Input: part model. Units: mm. Frame: model coordinates. Face numbers are marked on the shaded views. A direction names the side the tool comes from. Coordinates: 2 decimals unless noted, no trailing zeros. Loops run counter-clockwise (first coordinate to the right, second up) from the corner with the lowest first, then second, coordinate; pieces in that order, holes last.
(1) Contact query for flat-ended pins moving along their axis: P1, Ø3, axis at y = -2.5, z = 17, coming from the -X side; P2, Ø0.8, axis at x = -23, z = 16.5, coming from the -Y side; P3, Ø5, axis at x = -8.5, z = 0, coming from the -Y side. Output: stop coordinate, or through.
(2) Section B-B, the plane x = -23. Return loops of the section in (y, z), then the cut area to 3 significant figures.
(3) Line query: L1, parallel to X at y = -4.5, z = -18.5; L2, parallel to Z at x = 0, y = 0.2; L3, parallel to Z at x = -12, y = -3.75. Output: solid intervals per line, ascending.
(4) Section D-D, the plane z = -8.5. Return loops of the section in (x, y), then the cut area to 3 significant figures.
(5) Section C-C, the plane y = -6.25. Return loops of the section in (x, z).
(6) Mould query, pull axis Z, two halves, no side actions, for the marked faces 1, 2 and 3. Classes: released by +Z, released by -Z, zero draft, split by the parting line, or undercut.
(7) Section A-A, the plane z = 17. Return loops of the section in (x, y).
(8) Set-up query: the marked faces 4 and 5. Return all of +Z, -Z, +X, -X, +Y, -Y with unobstructed straight access to the full face (end or side cutting, diameter ignored); none if empty.
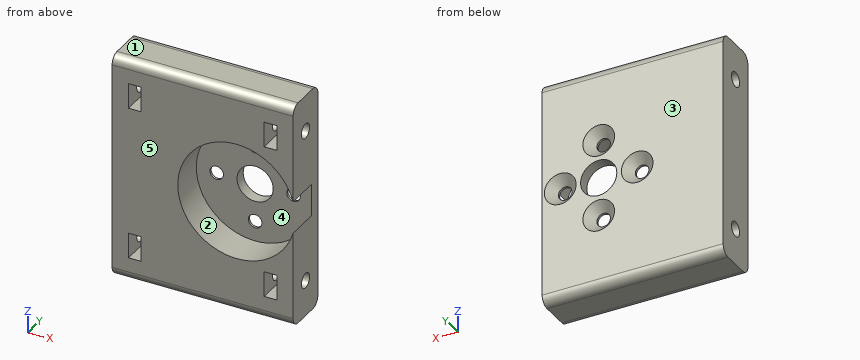
Autodesk Inventor part; units mm, degrees
ref_plane "YZ Plane" through (0, 0, 0) normal (1, 0, 0) x (0, 1, 0)
ref_plane "XZ Plane" through (0, 0, 0) normal (0, 1, 0) x (-1, 0, 0)
ref_plane "XY Plane" through (0, 0, 0) normal (0, 0, 1) x (1, 0, 0)
sketch "Эскиз1" plane through (0, 0, 0) normal (0, 1, 0) x (-1, 0, 0)
  circle A0 centre (0, 0) radius 12.5 construction
  circle A1 centre (0, 0) radius 8.5 construction
  circle A2 centre (8.5, 0) radius 1.5
  circle A3 centre (-8.5, 0) radius 1.5
  circle A4 centre (0, 0) radius 4
  line L0 (27.5, 25) -> (-12.5, 25)
  line L1 (-12.5, 25) -> (-12.5, -25)
  line L2 (-12.5, -25) -> (27.5, -25)
  line L3 (27.5, -25) -> (27.5, 25)
  line L4 (0, -12.5) -> (0, 12.5) construction
  line L5 (-12.5, 0) -> (12.5, 0) construction
  circle A5 centre (0, -8.5) radius 1.5
  circle A6 centre (0, 8.5) radius 1.5
  point P0 (7.5, 25)
  point P1 (7.5, -25)
  dimension "d0" = 25
  dimension "d1" = 17
  dimension "d2" = 3
  dimension "d3" = 3
  dimension "d4" = 8
  dimension "d5" = 40
  dimension "d6" = 50
  dimension "d7" = 25
  dimension "d26" = 25
  dimension "d31" = 90
  dimension "d32" = 90
  dimension "d33" = 3
  dimension "d34" = 3
extrude "Выдавливание1" add sketch "Эскиз1" along normal blind 2.5
sketch "Эскиз2" plane through (0, 0, 0) normal (0, -1, 0) x (1, 0, 0)
  circle A0 centre (0, 0) radius 13
  line L0 (12.5, 25) -> (12.5, -25)
  line L1 (-27.5, 25) -> (12.5, 25)
  line L2 (-27.5, -25) -> (-27.5, 25)
  line L3 (12.5, -25) -> (-27.5, -25)
  circle A1 centre (-8.5, 0) radius 1.5
  circle A2 centre (8.5, 0) radius 1.5
  circle A3 centre (0, 0) radius 4
  point P0 (12.5, -3.5707)
  point P1 (12.5, 3.5707)
  dimension "d10" = 26
extrude "Выдавливание2" add sketch "Эскиз2" along normal blind 7.5 contours A0 L0 L3 L2 L1
fillet "Сопряжение1" radius 2 4 edges at (-7.5, -7.5, -25) (-7.5, 2.5, -25) (-7.5, -7.5, 25) (-7.5, 2.5, 25)
sketch "Эскиз4" plane through (-27.5, -5.5, -25) normal (-1, 0, 0) x (0, 0, 1)
  arc A0 (50, 6) -> (48, 8) centre (48, 6) ccw
  line L0 (2, 8) -> (48, 8)
  arc A1 (2, 8) -> (0, 6) centre (2, 6) ccw
  line L1 (0, 0) -> (0, 6)
  arc A2 (0, 0) -> (2, -2) centre (2, 0) ccw
  line L2 (48, -2) -> (2, -2)
  arc A3 (48, -2) -> (50, 0) centre (48, 0) ccw
  line L3 (50, 0) -> (50, 6)
  circle A4 centre (42, 3) radius 1.65
  circle A5 centre (8, 3) radius 1.65
  point P0 (25, 5.5)
  point P1 (50, 3)
  dimension "d21" = 3.3
  dimension "d22" = 3.3
  dimension "d41" = 5
  dimension "d42" = 34
  dimension "d43" = 8
  dimension "d44" = 5
extrude "Выдавливание4" cut sketch "Эскиз4" against normal through all contours A4 | A5
chamfer "Фаска1" distance 2 angle 45 4 edges at (-7, 2.5, 0) (10, 2.5, 0) (1.5, 2.5, -8.5) (1.5, 2.5, 8.5)
sketch "Эскиз5" plane through (0, -7.5, 0) normal (0, -1, 0) x (1, 0, 0)
  line L0 (-27.5, 23) -> (12.5, 23)
  line L1 (-27.5, 23) -> (-27.5, -23)
  line L2 (12.5, -23) -> (-27.5, -23)
  line L3 (12.5, -23) -> (12.5, -3.5707)
  arc A0 (12.5, 3.5707) -> (12.5, -3.5707) centre (0, 0) ccw
  line L4 (12.5, 3.5707) -> (12.5, 23)
  line L5 (-27.5, -18.65) -> (12.5, -18.65)
  line L6 (-27.5, -15.35) -> (12.5, -15.35)
  line L7 (12.5, -18.65) -> (12.5, -15.35)
  line L8 (12.5, -17) -> (-27.5, -17) construction
  line L9 (8.9, -14.2) -> (6.1, -14.2)
  line L10 (6.1, -14.2) -> (6.1, -19.8)
  line L11 (6.1, -19.8) -> (8.9, -19.8)
  line L12 (8.9, -19.8) -> (8.9, -14.2)
  line L13 (8.9, -14.2) -> (6.1, -19.8) construction
  line L14 (6.1, -14.2) -> (8.9, -19.8) construction
  circle A1 centre (0, 0) radius 4
  line L15 (0, 0) -> (12.5, 0) construction
  line L16 (12.5, 3.5707) -> (12.5, -3.5707)
  line L17 (-7.5, -23) -> (-7.5, 23) construction
  line L18 (8.9, 14.2) -> (6.1, 14.2)
  line L19 (6.1, 14.2) -> (6.1, 19.8)
  line L20 (6.1, 19.8) -> (8.9, 19.8)
  line L21 (8.9, 19.8) -> (8.9, 14.2)
  line L22 (8.9, 14.2) -> (6.1, 19.8) construction
  line L23 (6.1, 14.2) -> (8.9, 19.8) construction
  line L24 (-23.9, -14.2) -> (-21.1, -14.2)
  line L25 (-21.1, -14.2) -> (-21.1, -19.8)
  line L26 (-21.1, -19.8) -> (-23.9, -19.8)
  line L27 (-23.9, -19.8) -> (-23.9, -14.2)
  line L28 (-23.9, -14.2) -> (-21.1, -19.8) construction
  line L29 (-21.1, -14.2) -> (-23.9, -19.8) construction
  line L30 (-21.1, 14.2) -> (-21.1, 19.8)
  line L31 (-21.1, 19.8) -> (-23.9, 19.8)
  line L32 (-23.9, 14.2) -> (-21.1, 14.2)
  line L33 (-23.9, 19.8) -> (-23.9, 14.2)
  line L34 (-23.9, 14.2) -> (-21.1, 19.8) construction
  line L35 (-21.1, 14.2) -> (-23.9, 19.8) construction
  point P0 (7.5, -17)
  point P1 (12.5, -13.2854)
  point P2 (7.5, 17)
  point P3 (-22.5, -17)
  point P4 (-22.5, 17)
  dimension "d35" = 2.8
  dimension "d36" = 5.6
  dimension "d38" = 5
extrude "Выдавливание5" cut sketch "Эскиз5" against normal blind 8.5 contours L27 L24 L25 L6 | L6 L25 L5 L27 | L5 L25 L26 L27 | L10 L9 L12 L6 | L6 L12 L5 L10 | L5 L12 L11 L10 | L18 L19 L20 L21 | L32 L33 L31 L30
equation "\"d22\" = d21"
properties part number "motoramma_1"
Report:
1. P1: passes through
1. P2: stops at y = 1
1. P3: stops at y = 0
2. outline: (-7.5, -23) arc R2 ccw to (-5.5, -25) - (0.5, -25) arc R2 ccw to (2.5, -23) - (2.5, 23) arc R2 ccw to (0.5, 25) - (-5.5, 25) arc R2 ccw to (-7.5, 23) - (-7.5, 19.8) - (1, 19.8) - (1, 14.2) - (-7.5, 14.2) - (-7.5, -14.2) - (1, -14.2) - (1, -19.8) - (-7.5, -19.8) - close
2. area: 401 mm2
3. L1: x = -27.5 to -23.9, -21.1 to 6.1, 8.9 to 12.5
3. L2: z = -25 to -10, -7 to -4, 4 to 7, 10 to 25
3. L3: z = -25 to -18.08, -15.92 to -5, 5 to 15.92, 18.08 to 25
4. outline: (-27.5, -7.5) - (-9.84, -7.5) - (-9.84, 0) - (-1.5, 0) - (-1.5, 0.5) - (-3.5, 2.5) - (-27.5, 2.5) - close; (1.5, 0) - (9.84, 0) - (9.84, -7.5) - (12.5, -7.5) - (12.5, 2.5) - (3.5, 2.5) - (1.5, 0.5) - close
4. area: 241 mm2
5. outline: (-27.5, -24.85) - (12.5, -24.85) - (12.5, -3.57) arc R13 cw (long way) to (12.5, 3.57) - (12.5, 24.85) - (-27.5, 24.85) - close; hole (-23.9, -19.8) - (-21.1, -19.8) - (-21.1, -14.2) - (-23.9, -14.2) - close; hole (-23.9, 14.2) - (-21.1, 14.2) - (-21.1, 19.8) - (-23.9, 19.8) - close; hole (6.1, -19.8) - (8.9, -19.8) - (8.9, -14.2) - (6.1, -14.2) - close; hole (6.1, 14.2) - (8.9, 14.2) - (8.9, 19.8) - (6.1, 19.8) - close
6. face 1: released by +Z
6. face 2: undercut
6. face 3: zero draft
7. outline: (-27.5, -7.5) - (-23.9, -7.5) - (-23.9, -4.15) - (-27.5, -4.15) - close; (-27.5, -0.85) - (-23.9, -0.85) - (-23.9, 1) - (-21.1, 1) - (-21.1, -0.85) - (6.1, -0.85) - (6.1, 1) - (8.9, 1) - (8.9, -0.85) - (12.5, -0.85) - (12.5, 2.5) - (-27.5, 2.5) - close; (-21.1, -7.5) - (6.1, -7.5) - (6.1, -4.15) - (-21.1, -4.15) - close; (8.9, -7.5) - (12.5, -7.5) - (12.5, -4.15) - (8.9, -4.15) - close
8. face 4: -Y
8. face 5: +Z, -Z, +X, -X, -Y
